Could you check a few things on this model? Use its own coordinates, in mm. A direction names the side the tool comes from. Coordinates: 2 decimals unless noted, no trailing zeros. Write each loop counter-clockwise with the first axis right and the second up, starting at its lowest first coordinate (ties: lowest second). Pieces come first, ordered by that corner, then holes. Notation, with made-up numbers: (23.25, 24.5) - (76.25, 24.5) arc R31 ccw to (76.25, 51.5) - close; hole circle Ø5 at (-17.5, 4). An arc over 180 degrees is marked (long way). Answer as a JSON object with one key per item and string values. Group by question number.
1) If we section it at D-D (y = 17.5): Write out the boundary of the cut face in (x, z).
2) Please list where these lines run through material, in increasing order: line 1 along X through (y, z) = (36.1, 15); line 2 along Z through (x, y) = (-20, 36); line 3 along Z through (x, y) = (-19.5, 37.5).
3) If we section it at A-A (z = 29.5): Write out the boundary of the cut face in (x, y).
4) If we section it at C-C (y = -3): Write out the boundary of the cut face in (x, z).
5) Will these pins go through, and if not, where does the flat tip stop? pin 1 Ø1 at (y, z) = (29.5, 29.5) entering from -X; pin 2 Ø1.5 at (x, y) = (-8.5, 35) entering from -Z; pin 3 Ø1.4 at (x, z) = (-41, 37) entering from -Y.
6) We'd pull the mould along Z, two halves only. Please class faces 1 (the cylindrical face through (-13.255, 36.014, 60.172)), 2 (the flat face through (-20, 35, 23)), 3 (the cylindrical face through (-27.493, -3.472, 14.67)), 4 (the flat face through (-40.99, 29.24, 33.75)): released by +Z, released by -Z, zero draft, split by the parting line, or undercut.
7) On a 3-axis mill with a long thin cutter (end or side, diameter ignored), from which of +Z, -Z, +X, -X, +Y, -Y can I reach the whole of each face in a straight line? I mean faces 5 (the flat face through (-40.99, 29.27, 36.22)), 6 (the flat face through (-41, 20, 36.233)), 7 (the flat face through (-20, 35, 63)). Say none if no direction works.
8) If we section it at B-B (x = -4): Write out the boundary of the cut face in (y, z), plus the area to 3 significant figures.
```python
from build123d import *

# Parameters (mm, degrees)
SKETCH1_W           = 40
SKETCH1_H           = 40
SKETCH1_W_2         = 34
SKETCH1_H_2         = 34
BOSS_EXTRUDE1_DEPTH = 70
SKETCH2_W           = 34
SKETCH2_H           = 3
BOSS_EXTRUDE2_DEPTH = 37
CUT_EXTRUDE1_DEPTH  = 37
SKETCH4_R           = 8.5
SKETCH4_R_2         = 7.5
BOSS_EXTRUDE3_DEPTH = 2
SKETCH6_R           = 7.5
BOSS_EXTRUDE4_DEPTH = 10
FILLET2_R           = 1.5
FILLET3_R           = 1.5
FILLET4_R           = 1.5
FILLET5_R           = 1.5
BOSS_EXTRUDE5_DEPTH = 2


with BuildPart() as part:
    # Sketch1 → Boss-Extrude1 (new body)
    with BuildSketch(Plane.XY):
        with Locations((-20, 20)):
            Rectangle(SKETCH1_W, SKETCH1_H)
        with Locations((-20, 20)):
            Rectangle(SKETCH1_W_2, SKETCH1_H_2, mode=Mode.SUBTRACT)
    extrude(amount=BOSS_EXTRUDE1_DEPTH)

    # Sketch2 → Boss-Extrude2 (add)
    with BuildSketch(Plane(origin=(0, 37, 0), x_dir=(-1, 0, 0), z_dir=(0, -1, 0))):
        with Locations((20, -68.5)):
            Rectangle(SKETCH2_W, SKETCH2_H)
    extrude(amount=BOSS_EXTRUDE2_DEPTH)

    # Sketch3 → Cut-Extrude1 (cut)
    with BuildSketch(Plane(origin=(0, 40, 0), x_dir=(1, 0, 0), z_dir=(0, 1, 0))):
        with BuildLine():
            ThreePointArc((-12.5, -15), (-14.696699141, -9.696699141), (-20, -7.5))
            Line((-20, -7.5), (-20, -15))
            Line((-20, -15), (-12.5, -15))
        make_face()
        with BuildLine():
            Line((-20, -15), (-20, -7.5))
            ThreePointArc((-20, -7.5), (-25.303300859, -9.696699141), (-27.5, -15))
            Line((-27.5, -15), (-20, -15))
        make_face()
        with BuildLine():
            Line((-12.5, -15), (-20, -15))
            Line((-20, -15), (-20, -22.5))
            ThreePointArc((-20, -22.5), (-14.696699141, -20.303300859), (-12.5, -15))
        make_face()
        with BuildLine():
            Line((-20, -22.5), (-20, -15))
            Line((-20, -15), (-27.5, -15))
            ThreePointArc((-27.5, -15), (-25.303300859, -20.303300859), (-20, -22.5))
        make_face()
        with BuildLine():
            ThreePointArc((-12.5, -55), (-14.696699141, -49.696699141), (-20, -47.5))
            Line((-20, -47.5), (-20, -55))
            Line((-20, -55), (-12.5, -55))
        make_face()
        with BuildLine():
            Line((-20, -55), (-20, -47.5))
            ThreePointArc((-20, -47.5), (-25.303300859, -49.696699141), (-27.5, -55))
            Line((-27.5, -55), (-20, -55))
        make_face()
        with BuildLine():
            Line((-12.5, -55), (-20, -55))
            Line((-20, -55), (-20, -62.5))
            ThreePointArc((-20, -62.5), (-14.696699141, -60.303300859), (-12.5, -55))
        make_face()
        with BuildLine():
            Line((-20, -62.5), (-20, -55))
            Line((-20, -55), (-27.5, -55))
            ThreePointArc((-27.5, -55), (-25.303300859, -60.303300859), (-20, -62.5))
        make_face()
    extrude(amount=-CUT_EXTRUDE1_DEPTH, mode=Mode.SUBTRACT)

    # Sketch4 → Boss-Extrude3 (add)
    with BuildSketch(Plane(origin=(0, 37, 0), x_dir=(-1, 0, 0), z_dir=(0, -1, 0))):
        with Locations((20, -15)):
            Circle(SKETCH4_R)
        with Locations((20, -15)):
            Circle(SKETCH4_R_2, mode=Mode.SUBTRACT)
        with Locations((20, -55)):
            Circle(SKETCH4_R)
        with Locations((20, -55)):
            Circle(SKETCH4_R_2, mode=Mode.SUBTRACT)
    extrude(amount=BOSS_EXTRUDE3_DEPTH)

    # Sketch6 → Boss-Extrude4 (add)
    with BuildSketch(Plane(origin=(0, 3, 0), x_dir=(1, 0, 0), z_dir=(0, 1, 0))):
        with Locations((-20, -15)):
            Circle(SKETCH6_R)
        with Locations((-20, -55)):
            Circle(SKETCH6_R)
    extrude(amount=-BOSS_EXTRUDE4_DEPTH)

    # Fillet2
    fillet2_edges = [part.edges().sort_by_distance(p)[0] for p in [
        (-27.5, -7, 55),
    ]]
    fillet(fillet2_edges, radius=FILLET2_R)

    # Fillet3
    fillet3_edges = [part.edges().sort_by_distance(p)[0] for p in [
        (-27.5, -7, 15),
    ]]
    fillet(fillet3_edges, radius=FILLET3_R)

    # Fillet4
    fillet4_edges = [part.edges().sort_by_distance(p)[0] for p in [
        (-27.5, 0, 15),
    ]]
    fillet(fillet4_edges, radius=FILLET4_R)

    # Fillet5
    fillet5_edges = [part.edges().sort_by_distance(p)[0] for p in [
        (-27.5, 0, 55),
    ]]
    fillet(fillet5_edges, radius=FILLET5_R)

    # Sketch9 → Boss-Extrude5 (add)
    with BuildSketch(Plane.ZY.offset(40)):
        Polygon((35, 30.488163829), (37.465362362, 28.022801468), (36.232681181, 28.022801468), (36.232681181, 12.265663865), (33.412251244, 12.265663865), (33.412251244, 28.022801468), (32.534637638, 28.022801468), align=None)
    extrude(amount=BOSS_EXTRUDE5_DEPTH)


solid = part.part
```
Here are the results:
{
 "1": {"outline": "(-42, 33.41) - (-40, 33.41) - (-40, 0) - (-37, 0) - (-37, 67) - (-3, 67) - (-3, 0) - (0, 0) - (0, 70) - (-40, 70) - (-40, 36.23) - (-42, 36.23) - close"},
 "2": {"line 1": "x = -40 to -37, -28.5 to -27.5, -12.5 to -11.5, -3 to 0", "line 2": "z = 6.5 to 7.5, 22.5 to 23.5, 46.5 to 47.5, 62.5 to 63.5, 67 to 70", "line 3": "z = 0 to 7.52, 22.48 to 47.52, 62.48 to 70"},
 "3": {"outline": "(-40, 0) - (0, 0) - (0, 40) - (-40, 40) - close; hole (-37, 3) - (-3, 3) - (-3, 37) - (-37, 37) - close"},
 "4": {"outline": "circle Ø15 at (-20, 15); circle Ø15 at (-20, 55)"},
 "5": {"pin 1": "stops at x = -40", "pin 2": "stops at z = 67", "pin 3": "stops at y = 28.02"},
 "6": {"face 1": "undercut", "face 2": "zero draft", "face 3": "undercut", "face 4": "released by -Z"},
 "7": {"face 5": "+Z, -X, +Y", "face 6": "+Z, -X, -Y", "face 7": "-Z"},
 "8": {"outline": "(0, 0) - (3, 0) - (3, 67) - (37, 67) - (37, 0) - (40, 0) - (40, 70) - (0, 70) - close", "area": "522 mm²"}
}
